Build history of the part. All positions in model axes, mm. Face numbers are marked on the shaded views. A direction names the side the tool comes from. Round coordinates to 2 decimals unless told otherwise and drop trailing zeros. Loops run counter-clockwise (first coordinate to the right, second up) from the corner with the lowest first, then second, coordinate; pieces in that order, holes last. Notation, with made-up numbers: (-9.75, 47.5) - (2.25, 47.5) arc R25 cw to (2.25, 79.5) - close; hole circle Ø1 at (-8, 82). An arc over 180 degrees is marked (long way). Put each result on its own line as item: value. Start each with the question number.
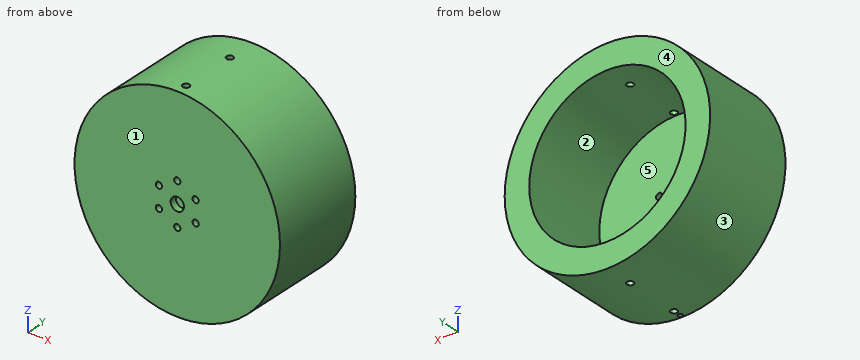
from build123d import *

# Parameters (mm, degrees)
SKETCH1_R               = 46
SKETCH1_R_2             = 3
SKETCH1_R_3             = 1.4
BOSS_EXTRUDE1_DEPTH     = 3
SKETCH6_R               = 1
CUT_EXTRUDE2_DEPTH      = 3
SKETCH7_R               = 46
SKETCH7_R_2             = 35
BOSS_EXTRUDE2_DEPTH     = 40
SKETCH8_R               = 1.5
CUT_EXTRUDE3_DEPTH      = 108
SKETCH9_R               = 1.5
CUT_EXTRUDE4_DEPTH      = 47.00000011
CUT_EXTRUDE4_DEPTH_BACK = 47.00000011


with BuildPart() as part:
    # Sketch1 → Boss-Extrude1 (new body)
    with BuildSketch(Plane(origin=(0, 0, 0), x_dir=(1, 0, 0), z_dir=(0, 1, 0))):
        Circle(SKETCH1_R)
        Circle(SKETCH1_R_2, mode=Mode.SUBTRACT)
        with Locations((0, 9.5)):
            Circle(SKETCH1_R_3, mode=Mode.SUBTRACT)
        with Locations((8.227241336, 4.75)):
            Circle(SKETCH1_R_3, mode=Mode.SUBTRACT)
        with Locations((8.227241336, -4.75)):
            Circle(SKETCH1_R_3, mode=Mode.SUBTRACT)
        with Locations((0, -9.5)):
            Circle(SKETCH1_R_3, mode=Mode.SUBTRACT)
        with Locations((-8.227241336, -4.75)):
            Circle(SKETCH1_R_3, mode=Mode.SUBTRACT)
        with Locations((-8.227241336, 4.75)):
            Circle(SKETCH1_R_3, mode=Mode.SUBTRACT)
    extrude(amount=BOSS_EXTRUDE1_DEPTH)

    # Sketch6 → Cut-Extrude2 (cut)
    with BuildSketch(Plane.XY.offset(-46)):
        with Locations((0, 1.5)):
            Circle(SKETCH6_R)
    extrude(amount=CUT_EXTRUDE2_DEPTH, mode=Mode.SUBTRACT)

    # Sketch7 → Boss-Extrude2 (add)
    with BuildSketch(Plane(origin=(0, 3, 0), x_dir=(1, 0, 0), z_dir=(0, 1, 0))):
        Circle(SKETCH7_R)
        Circle(SKETCH7_R_2, mode=Mode.SUBTRACT)
    extrude(amount=BOSS_EXTRUDE2_DEPTH)

    # Sketch8 → Cut-Extrude3 (cut)
    with BuildSketch(Plane.XY.offset(46)):
        with Locations((0, 30)):
            Circle(SKETCH8_R)
    extrude(amount=-CUT_EXTRUDE3_DEPTH, mode=Mode.SUBTRACT)

    # Sketch9 → Cut-Extrude4 (cut, two sides)
    with BuildSketch(Plane.XY) as cut_extrude4_sk:
        with Locations((0, 5)):
            Circle(SKETCH9_R)
    extrude(amount=CUT_EXTRUDE4_DEPTH, mode=Mode.SUBTRACT)
    extrude(cut_extrude4_sk.sketch, amount=-CUT_EXTRUDE4_DEPTH_BACK, mode=Mode.SUBTRACT)


solid = part.part
Item 1: Drill centre lines: probe 1 along Y at (x, z) = (0, -40.75); probe 2 along X at (y, z) = (2, 0); probe 3 along X at (y, z) = (1, 4). Where is each one in solid material? Low to high. Write a range as [from, to].
Item 2: Two-plate mould, pull along X, no slides. Class the marked faces 3, 4 and 5: pulls with the +X half, pulls with the -X half, needs draft (parallel to the pull), parting line crosses it, or undercut.
Item 3: Slice it at A-A (z = 0). Give the cut face in (x, y), plus the area to 3 significant figures.
Item 4: Slice it at B-B (x = -17). Give the cut face in (y, z), plus the area to 3 significant figures.
Item 5: Drop flat-ended pins along their axis: pin 1 Ø1.6 at (x, y) = (-0.5, 1.5) entering from -Z; pin 2 Ø1.5 at (y, z) = (37.5, 11) entering from +X; pin 3 Ø12 at (x, z) = (26, -36) entering from -Y; pin 4 Ø1.6 at (x, y) = (0, 1.5) entering from -Z. Give the stop position or say it passes through.
Item 6: Slice it at D-D (y = 9). Give the cut face in (x, z).
Item 7: Slice it at C-C (z = 21). Give the cut face in (x, y).
Item 8: Which spindle directions (+Z, -Z, +X, -X, +Y, -Y) get a long thin tool onto all of the face, cutting with end or side? Do the marked faces 1 and 2. Say none if no direction does.
Computed values:
1. probe 1: y = [0, 3.5], [6.5, 28.5], [31.5, 43]
1. probe 2: x = [-46, -3], [3, 46]
1. probe 3: x = [-45.83, -9.41], [-7.05, 7.05], [9.41, 45.83]
2. face 3: parting line crosses it
2. face 4: needs draft
2. face 5: undercut
3. outline: (-46, 0) - (-3, 0) - (-3, 3) - (-35, 3) - (-35, 43) - (-46, 43) - close; (3, 0) - (46, 0) - (46, 43) - (35, 43) - (35, 3) - (3, 3) - close
3. area: 1,140 mm^2
4. outline: (0, -42.74) - (43, -42.74) - (43, -30.59) - (3, -30.59) - (3, 30.59) - (43, 30.59) - (43, 42.74) - (0, 42.74) - close
4. area: 1,230 mm^2
5. pin 1: stops at z = -46
5. pin 2: stops at x = 44.84
5. pin 3: stops at y = 0
5. pin 4: stops at z = -43
6. outline: circle Ø92 at (0, 0); hole circle Ø70 at (0, 0)
7. outline: (-40.93, 0) - (40.93, 0) - (40.93, 43) - (28, 43) - (28, 3) - (-28, 3) - (-28, 43) - (-40.93, 43) - close
8. face 1: +Z, -Z, +X, -X, -Y
8. face 2: +Y
